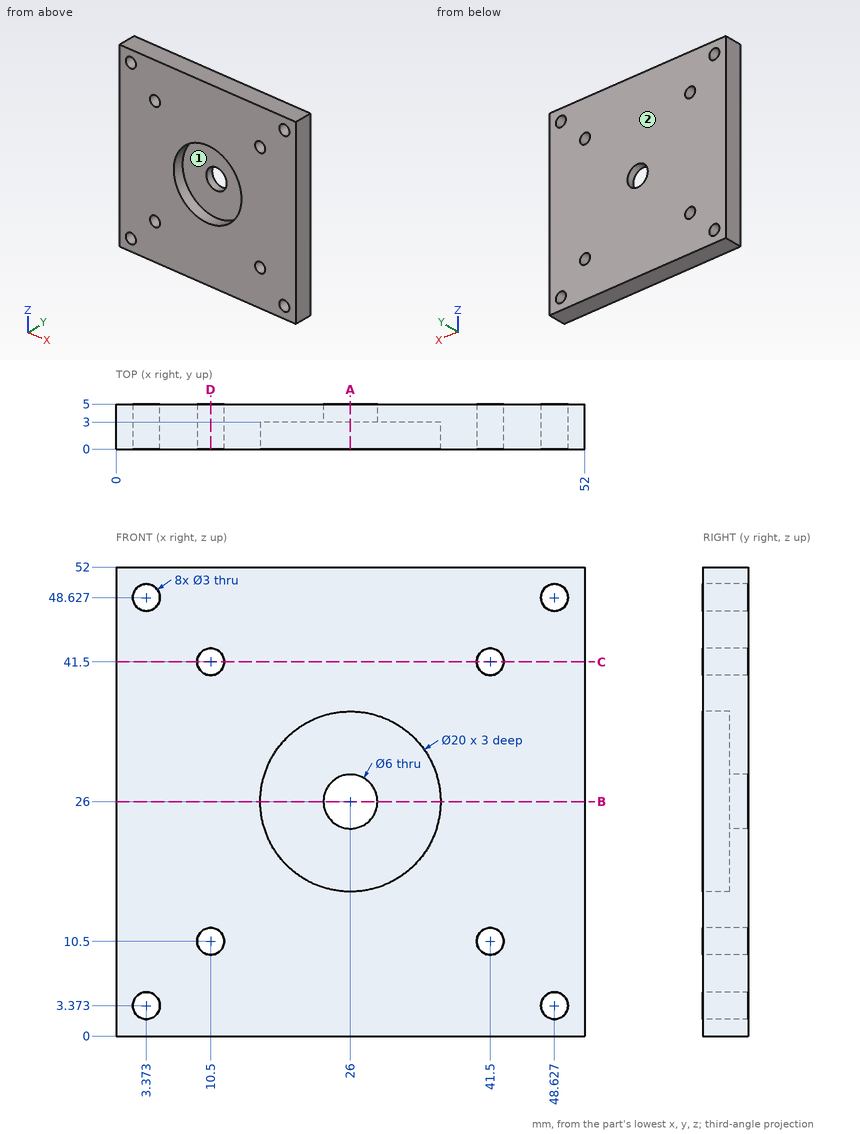
Could you check a few things on this drawing? It's one solid part, dimensions in mm from its lowest x, y, z. Coordinates: 2 decimals unless noted, no trailing zeros. Order: outer loops, then holes, each group sorted by start corner. A loop starts at its lowest first (then second) coordinate and runs counter-clockwise, first axis right, second up. Notation, with made-up numbers: M -0.5,-13.75 L 36.5,-13.75 A18 cw 36.5,13.25 Z; hole C 64,39 d2. An arc over 180 degrees is marked long. Answer as CSV lines item,"result".
(1) Please list where these lines run through material, in increasing order: L1, parallel to Z at x = 41.5, y = 1.85; L2, parallel to X at y = 1.6, z = 2 (1 decimal).
Geometry check:
L1,"0 to 9, 12 to 40, 43 to 52"
L2,"0 to 2.8, 4 to 48, 49.2 to 52"
(2) I'm going to push flat-ended pins straight in: pin 1 (1.8 mm diameter, centred on x = 48.63, z = 48.63, fed in from +Y); pin 2 (8 mm diameter, centred on x = 27, z = 22, fed in from -Y). Where does each tip first touch, or does it pass through?
Geometry check:
pin 1,"through"
pin 2,"y = 3"
(3) Suppose I cut it at A-A on x = 26. Please give me the cut outline in (y, z).
Geometry check:
outline,"M 0,0 L 5,0 L 5,23 L 3,23 L 3,16 L 0,16 Z; M 0,36 L 3,36 L 3,29 L 5,29 L 5,52 L 0,52 Z"
(4) If we mould it in two halves opening along X, with no side actions, what happens to the marked faces 1 and 2? For each: released by +X, released by -X, zero draft, split by the parting line, or undercut.
Geometry check:
face 1,"undercut"
face 2,"zero draft"
(5) Suppose I cut it at B-B on z = 26. Please give me the cut outline in (x, y), plus the area to 3 significant figures.
Geometry check:
outline,"M 0,0 L 16,0 L 16,3 L 23,3 L 23,5 L 0,5 Z; M 29,3 L 36,3 L 36,0 L 52,0 L 52,5 L 29,5 Z"
area,"188 mm^2"
(6) Suppose I cut it at D-D on x = 10.5. Please give me the cut outline in (y, z).
Geometry check:
outline,"M 0,0 L 5,0 L 5,9 L 0,9 Z; M 0,12 L 5,12 L 5,40 L 0,40 Z; M 0,43 L 5,43 L 5,52 L 0,52 Z"
(7) Suppose I cut it at C-C on z = 41.5. Please give me the cut outline in (x, y), plus the area to 3 significant figures.
Geometry check:
outline,"M 0,0 L 9,0 L 9,5 L 0,5 Z; M 12,0 L 40,0 L 40,5 L 12,5 Z; M 43,0 L 52,0 L 52,5 L 43,5 Z"
area,"230 mm^2"
